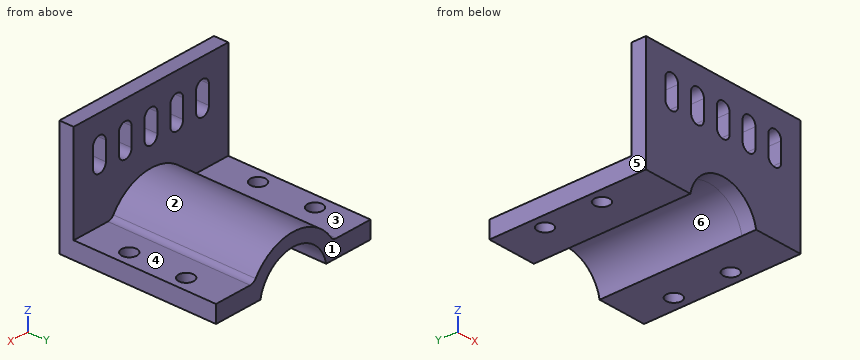
Autodesk Inventor part; units mm, degrees
ref_plane "YZ Plane" through (0, 0, 0) normal (1, 0, 0) x (0, 1, 0)
ref_plane "XZ Plane" through (0, 0, 0) normal (0, 1, 0) x (-1, 0, 0)
ref_plane "XY Plane" through (0, 0, 0) normal (0, 0, 1) x (1, 0, 0)
sketch "Sketch1" plane through (0, 0, 0) normal (0, 1, 0) x (-1, 0, 0)
  line L0 (0, 0) -> (-76.2, 0)
  line L1 (-76.2, 0) -> (-76.2, -50.8)
  line L2 (-76.2, -50.8) -> (0, -50.8)
  line L3 (0, -50.8) -> (0, 0)
  line L4 (-12.7, -11.7475) -> (-12.7, -20.0025) construction
  line L5 (-15.875, -11.7475) -> (-15.875, -20.0025)
  line L6 (-9.525, -20.0025) -> (-9.525, -11.7475)
  arc A0 (-9.525, -11.7475) -> (-15.875, -11.7475) centre (-12.7, -11.7475) ccw
  arc A1 (-15.875, -20.0025) -> (-9.525, -20.0025) centre (-12.7, -20.0025) ccw
  line L7 (-25.4, -11.7475) -> (-25.4, -20.0025) construction
  line L8 (-28.575, -11.7475) -> (-28.575, -20.0025)
  line L9 (-22.225, -20.0025) -> (-22.225, -11.7475)
  arc A2 (-22.225, -11.7475) -> (-28.575, -11.7475) centre (-25.4, -11.7475) ccw
  arc A3 (-28.575, -20.0025) -> (-22.225, -20.0025) centre (-25.4, -20.0025) ccw
  line L10 (-28.575, -11.7475) -> (-28.575, -20.0025)
  line L11 (-25.4, -11.7475) -> (-25.4, -20.0025) construction
  arc A4 (-22.225, -11.7475) -> (-28.575, -11.7475) centre (-25.4, -11.7475) ccw
  line L12 (-22.225, -20.0025) -> (-22.225, -11.7475)
  arc A5 (-28.575, -20.0025) -> (-22.225, -20.0025) centre (-25.4, -20.0025) ccw
  line L13 (-41.275, -11.7475) -> (-41.275, -20.0025)
  line L14 (-38.1, -11.7475) -> (-38.1, -20.0025) construction
  arc A6 (-34.925, -11.7475) -> (-41.275, -11.7475) centre (-38.1, -11.7475) ccw
  line L15 (-34.925, -20.0025) -> (-34.925, -11.7475)
  arc A7 (-41.275, -20.0025) -> (-34.925, -20.0025) centre (-38.1, -20.0025) ccw
  line L16 (-53.975, -11.7475) -> (-53.975, -20.0025)
  line L17 (-50.8, -11.7475) -> (-50.8, -20.0025) construction
  arc A8 (-47.625, -11.7475) -> (-53.975, -11.7475) centre (-50.8, -11.7475) ccw
  line L18 (-47.625, -20.0025) -> (-47.625, -11.7475)
  arc A9 (-53.975, -20.0025) -> (-47.625, -20.0025) centre (-50.8, -20.0025) ccw
  line L19 (-66.675, -11.7475) -> (-66.675, -20.0025)
  line L20 (-63.5, -11.7475) -> (-63.5, -20.0025) construction
  arc A10 (-60.325, -11.7475) -> (-66.675, -11.7475) centre (-63.5, -11.7475) ccw
  line L21 (-60.325, -20.0025) -> (-60.325, -11.7475)
  arc A11 (-66.675, -20.0025) -> (-60.325, -20.0025) centre (-63.5, -20.0025) ccw
  point P0 (-12.7, -15.875)
  point P1 (-25.4, -15.875)
  point P2 (-25.4, -15.875)
  point P3 (-38.1, -15.875)
  point P4 (-50.8, -15.875)
  point P5 (-63.5, -15.875)
  dimension "d0" = 50.8
  dimension "d1" = 76.2
  dimension "d41" = 8.255
  dimension "d42" = 6.35
  dimension "d43" = 12.7
  dimension "d44" = 8.255
  dimension "d45" = 6.35
  dimension "d56" = 12.7
  dimension "d57" = 15.875
  dimension "d60" = 12.7
extrude "Extrusion1" add sketch "Sketch1" along normal blind 6.35
sketch "Sketch2" plane through (0, 6.35, 0) normal (0, 1, 0) x (1, 0, 0)
  line L0 (76.2, 50.8) -> (0, 50.8)
  circle A0 centre (38.1, 53.975) radius 16.51
  line L1 (0, 50.8) -> (0, 0)
  circle A1 centre (38.1, 53.975) radius 22.225
  line L2 (18.6727, 43.18) -> (0, 43.18)
  line L3 (76.2, 50.8) -> (0, 50.8)
  line L4 (57.5273, 43.18) -> (76.2, 43.18)
  line L5 (76.2, 0) -> (76.2, 50.8)
  point P0 (54.3018, 50.8)
  point P1 (21.8982, 50.8)
  dimension "d22" = 33.02
  dimension "d23" = 3.175
  dimension "d24" = 38.1
  dimension "d25" = 44.45
  dimension "d26" = 7.62
  dimension "d27" = 7.62
extrude "Extrusion2" add sketch "Sketch2" along normal blind 63.5 contours L5 L4 A1 L0 | A1 L0 A0 | L2 L1 L0 A1 picked at (21.7987, 42.02)
sketch "Sketch3" plane through (0, 6.35, -43.18) normal (0, 0, 1) x (1, 0, 0)
  line L0 (76.2, 0) -> (76.2, 63.5)
  line L1 (0, 0) -> (0, 63.5)
  line L2 (0, 63.5) -> (18.6727, 63.5)
  line L3 (57.5273, 63.5) -> (76.2, 63.5)
  line L4 (54.3018, 0) -> (21.8982, 0)
  point P0 (0, -6.35)
  point P1 (6.35, 44.45)
  point P2 (69.85, 44.45)
  point P3 (6.35, 19.05)
  point P4 (69.85, 19.05)
  dimension "d30" = 6.35
  dimension "d31" = 6.35
  dimension "d32" = 19.05
  dimension "d33" = 19.05
  dimension "d52" = 6.35
  dimension "d53" = 6.35
  dimension "d54" = 19.05
  dimension "d55" = 19.05
hole "Hole1" at (6.35, 50.8, -43.18) at (6.35, 25.4, -43.18) at (69.85, 25.4, -43.18) at (69.85, 50.8, -43.18) direction (0, 0, -1) diameter 6.7564 end through all
fillet "Fillet1" radius 3.175 2 edges at (18.6727, 38.1, -43.18) (57.5273, 38.1, -43.18)
sketch "Sketch6" plane through (0, 6.35, 0) normal (0, 1, 0) x (1, 0, 0)
  circle A0 centre (38.1, 53.975) radius 16.51
  arc A1 (21.8982, 50.8) -> (54.3018, 50.8) centre (38.1, 53.975) ccw
  point P0 (0, 0)
  dimension "d49" = 33.02
extrude "Extrusion3" cut sketch "Sketch6" against normal blind 25.4
properties part number "CLAMP"
CAD build for the part. Positions are in the model's coordinates, mm. Face numbers are marked on the shaded views. A direction names the side the tool comes from. Give positions to 0.01 mm unless a question says otherwise; leave off trailing zeros. Write each loop counter-clockwise with the first axis right and the second up, starting at its lowest first coordinate (ties: lowest second). Pieces come first, ordered by that corner, then holes. Notation, with made-up numbers: M 31,76 L 63,76 A14 cw 63,84 Z; hole C -25.5,61 d9. An arc over 180 degrees is marked long. Put each result on its own line as item: value. Start each with the question number.
(1) Probe L1, parallel to Y at x = 6.35, z = -49; L2, parallel to X at y = 50.8, z = -46; L3, parallel to Z at x = 9.5, y = 6.5. List the from-to ranges inside material, lowest first.
(2) Band-saw the part on D-D, the plane y = 25.4. Write the cut outline in (x, z) (3 decimals).
(3) Band-saw the part on A-A, the plane z = -18. Write the cut outline in (x, y) (3 decimals), and give its area (3 significant figures).
(4) Mould opens along X. For the marked faces 4, 5 and 6 say: +X half, -X half, draft (parallel to the pull), parting line (faces both ways), or undercut.
(5) Band-saw the part on C-C, the plane z = -44.5. Write the cut outline in (x, y), and give its area (3 significant figures).
(6) Band-saw the part on B-B, the plane x = 6.35. Write the cut outline in (y, z).
(7) Which spindle directions (+Z, -Z, +X, -X, +Y, -Y) get a long thin tool onto all of the face, cutting with end or side? Do the marked faces 1, 2 and 3. Say none if no direction does.
(8) Flat gauge pins, fed straight in: pin 1 Ø1.5 at (x, y) = (35.5, 41.5) entering from -Z; pin 2 Ø8 at (y, z) = (7.5, -28.5) entering from -X; pin 3 Ø11 at (x, y) = (69.85, 25.4) entering from +Z; pin 4 Ø18.5 at (x, y) = (67, 34) entering from +Z. Where does each tip first touch, or does it go through?
Response values:
1. L1: y = 0 to 22.02, 28.78 to 47.42, 54.18 to 69.85
1. L2: x = 0 to 2.97, 9.73 to 23.64, 52.56 to 66.47, 73.23 to 76.2
1. L3: z = -50.8 to -43.18
2. outline: M 0,-50.8 L 2.972,-50.8 L 2.972,-43.18 L 0,-43.18 Z; M 9.728,-50.8 L 21.898,-50.8 A16.51 cw 54.302,-50.8 L 66.472,-50.8 L 66.472,-43.18 L 59.313,-43.18 A3.175 cw 56.662,-41.751 A22.225 ccw 19.538,-41.751 A3.175 cw 16.887,-43.18 L 9.728,-43.18 Z; M 73.228,-50.8 L 76.2,-50.8 L 76.2,-43.18 L 73.228,-43.18 Z
3. outline: M 0,0 L 9.525,0 L 9.525,6.35 L 0,6.35 Z; M 15.875,0 L 22.225,0 L 22.225,6.35 L 15.875,6.35 Z; M 28.575,0 L 34.925,0 L 34.925,6.35 L 28.575,6.35 Z; M 41.275,0 L 47.625,0 L 47.625,6.35 L 41.275,6.35 Z; M 53.975,0 L 60.325,0 L 60.325,6.35 L 53.975,6.35 Z; M 66.675,0 L 76.2,0 L 76.2,6.35 L 66.675,6.35 Z
3. area: 282 mm2
4. face 4: draft
4. face 5: -X half
4. face 6: undercut
5. outline: M 0,0 L 24.58,0 L 24.58,69.85 L 0,69.85 Z; M 51.62,0 L 76.2,0 L 76.2,69.85 L 51.62,69.85 Z; hole C 6.35,25.4 d6.76; hole C 6.35,50.8 d6.76; hole C 69.85,25.4 d6.76; hole C 69.85,50.8 d6.76
5. area: 3,290 mm2
6. outline: M 0,-50.8 L 22.02,-50.8 L 22.02,-43.18 L 6.35,-43.18 L 6.35,0 L 0,0 Z; M 28.78,-50.8 L 47.42,-50.8 L 47.42,-43.18 L 28.78,-43.18 Z; M 54.18,-50.8 L 69.85,-50.8 L 69.85,-43.18 L 54.18,-43.18 Z
7. face 1: +Z, -Z, +X, -X, +Y
7. face 2: +Z, +Y
7. face 3: +Z, -X, +Y
8. pin 1: stops at z = -37.81
8. pin 2: stops at x = 0
8. pin 3: stops at z = -43.18
8. pin 4: stops at z = -42.77
